Work out the finished part from the listing and answer in its coordinate system (mm). A direction names the side the tool comes from. Round coordinates to 2 decimals unless told otherwise and drop trailing zeros. Write each loop counter-clockwise with the first axis right and the second up, starting at its lowest first coordinate (ties: lowest second). Pieces come first, ordered by that corner, then holes. Notation, with made-up numbers: (-23, 55.5) - (31, 55.5) arc R23 ccw to (31, 75.5) - close; hole circle Ø10 at (-31.5, -18). An arc over 180 degrees is marked (long way). Answer as a JSON object with one key per item and string values.
```python
from build123d import *

# Parameters (mm, degrees)
SKETCH1_R           = 2.75
BOSS_EXTRUDE1_DEPTH = 3
SKETCH2_W           = 65
SKETCH2_H           = 3
BOSS_EXTRUDE2_DEPTH = 35
SKETCH3_R           = 1.25
CUT_EXTRUDE1_DEPTH  = 4


with BuildPart() as part:
    # Sketch1 → Boss-Extrude1 (new body)
    with BuildSketch(Plane(origin=(0, 0, 0), x_dir=(1, 0, 0), z_dir=(0, 1, 0))):
        Polygon((0, 0), (16, 0), (16, 6), (49, 6), (49, 0), (65, 0), (65, 18), (0, 18), align=None)
        with Locations((7.69, 5)):
            Circle(SKETCH1_R, mode=Mode.SUBTRACT)
        with Locations((57.31, 5)):
            Circle(SKETCH1_R, mode=Mode.SUBTRACT)
    extrude(amount=BOSS_EXTRUDE1_DEPTH)

    # Sketch2 → Boss-Extrude2 (add)
    with BuildSketch(Plane(origin=(0, 0, 0), x_dir=(1, 0, 0), z_dir=(0, 1, 0))):
        with Locations((32.5, 19.5)):
            Rectangle(SKETCH2_W, SKETCH2_H)
    extrude(amount=BOSS_EXTRUDE2_DEPTH)

    # Sketch3 → Cut-Extrude1 (cut, through all)
    with BuildSketch(Plane.XY.offset(-18)):
        with Locations((16.5, 20.5)):
            Circle(SKETCH3_R)
        with Locations((48.5, 20.5)):
            Circle(SKETCH3_R)
    extrude(amount=-CUT_EXTRUDE1_DEPTH, mode=Mode.SUBTRACT)


solid = part.part
```
Item 1: Each of these flat-tipped pins is pushed along its axis until it touches: P1, Ø1, axis at x = 19.5, z = -12, coming from the -Y side; P2, Ø3, axis at x = 16.5, y = 20.5, coming from the +Z side; P3, Ø2.5, axis at x = 40.5, y = 2, coming from the +Z side; P4, Ø8, axis at y = 18.5, z = -12, coming from the -X side. Where does it stop, or does it pass through?
Results found:
{"P1": "y = 0", "P2": "z = -18", "P3": "z = -6", "P4": "through"}
Item 2: A cutting plane is placed at B-B (x = 7.69). Write down the section's boundary in (y, z), and give its area (4 significant figures).
Results found:
{"outline": "(0, -21) - (35, -21) - (35, -18) - (3, -18) - (3, -7.75) - (0, -7.75) - close; (0, -2.25) - (3, -2.25) - (3, 0) - (0, 0) - close", "area": "142.5 mm²"}
Item 3: A cutting plane is placed at D-D (x = 25). Write down the section's boundary in (y, z), and give its area (3 significant figures).
Results found:
{"outline": "(0, -21) - (35, -21) - (35, -18) - (3, -18) - (3, -6) - (0, -6) - close", "area": "141 mm²"}
Item 4: A cutting plane is placed at C-C (y = 20.5). Write down the section's boundary in (x, z), and give its area (3 significant figures).
Results found:
{"outline": "(0, -21) - (15.25, -21) - (15.25, -18) - (0, -18) - close; (17.75, -21) - (47.25, -21) - (47.25, -18) - (17.75, -18) - close; (49.75, -21) - (65, -21) - (65, -18) - (49.75, -18) - close", "area": "180 mm²"}
Item 5: For faces 1 (the flat face through (32, 19, -18)), 2 (the flat face through (57, 1, 0)), 3 (the flat face through (32, 1, -6)), determine the directions among +Z, -Z, +X, -X, +Y, -Y from which every point of the face is accessible in a straight line to the end or side of a thin tool.
Results found:
{"face 1": "+Z, +X, -X, +Y", "face 2": "+Z, +X, -X, +Y, -Y", "face 3": "+Z, +Y, -Y"}
Item 6: Consider line 1 along Z through (x, y) = (7.69, 1.45); line 2 along Y through (x, z) = (27.5, -12.5); line 3 along Z through (x, y) = (46, 13.5). Determine where each line is inside the solid, lowest interval first.
Results found:
{"line 1": "-21 to -7.75, -2.25 to 0", "line 2": "0 to 3", "line 3": "-21 to -18"}
Item 7: Determine the mould class of faces 4 (the cylindrical face through (48.23, 19.28, -19.48)), 5 (the flat face through (32, 35, -20)), 6 (the flat face through (8, 1, 0)) for opening direction Y: pulls with the +Y half, pulls with the -Y half, needs draft (parallel to the pull), parting line crosses it, or undercut.
Results found:
{"face 4": "undercut", "face 5": "pulls with the +Y half", "face 6": "needs draft"}
Item 8: A cutting plane is placed at A-A (z = -5). Write down the section's boundary in (x, y), and give its area (3 significant figures).
Results found:
{"outline": "(0, 0) - (4.94, 0) - (4.94, 3) - (0, 3) - close; (10.44, 0) - (16, 0) - (16, 3) - (10.44, 3) - close; (49, 0) - (54.56, 0) - (54.56, 3) - (49, 3) - close; (60.06, 0) - (65, 0) - (65, 3) - (60.06, 3) - close", "area": "63.0 mm²"}
